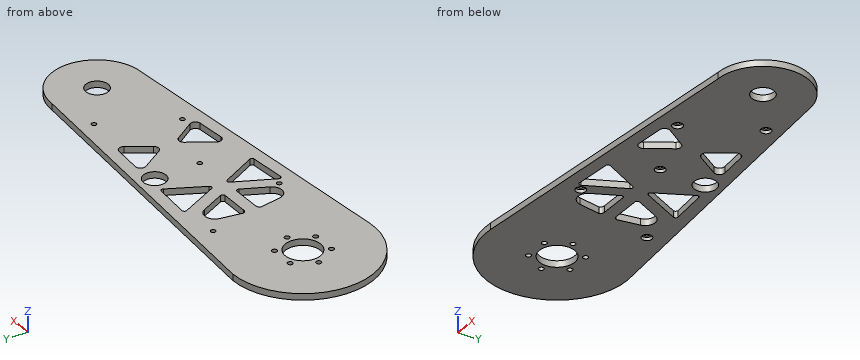
from build123d import *

# Parameters (mm, degrees)
SKETCH1_R              = 14.29385
SKETCH1_R_2            = 11.115
SKETCH1_R_3            = 11.1125
BOSS_EXTRUDE1_DEPTH    = 6.35
CROQUIS1_R             = 2.38125
CORTAR_EXTRUIR1_DEPTH  = 50
CROQUIS6_R             = 2.38125
CORTAR_EXTRUIR6_DEPTH  = 10
CROQUIS8_R             = 17.5
CORTAR_EXTRUIR8_DEPTH  = 10
CROQUIS9_R             = 2.5527
CORTAR_EXTRUIR9_DEPTH  = 10
CROQUIS5_R             = 2.38125
CORTAR_EXTRUIR5_DEPTH  = 10
CROQUIS10_R            = 5
CORTAR_EXTRUIR10_DEPTH = 3.18


with BuildPart() as part:
    # Sketch1 → Boss-Extrude1 (new body)
    with BuildSketch(Plane.XY):
        with BuildLine():
            Line((0, 70), (310, 45))
            ThreePointArc((310, 45), (355, 0), (310, -45))
            Line((310, -45), (5.171398252, -69.808714643))
            ThreePointArc((5.171398252, -69.808714643), (-69.952162315, -2.587467389), (0, 70))
        make_face()
        Circle(SKETCH1_R, mode=Mode.SUBTRACT)
        with Locations((310, 0)):
            Circle(SKETCH1_R_2, mode=Mode.SUBTRACT)
        with Locations((162.878542763, 40)):
            Circle(SKETCH1_R_3, mode=Mode.SUBTRACT)
        with BuildLine():
            Line((107.898974887, 49.259511156), (143.314248041, 46.40344074))
            ThreePointArc((143.314248041, 46.40344074), (145.093535791, 45.259647961), (145.131116366, 43.144768645))
            Line((145.131116366, 43.144768645), (127.657910713, 9.007596386))
            ThreePointArc((127.657910713, 9.007596386), (125.636568061, 7.786360797), (123.64194899, 9.050772613))
            Line((123.64194899, 9.050772613), (105.699881489, 46.044015288))
            ThreePointArc((105.699881489, 46.044015288), (105.866657482, 48.289689684), (107.898974887, 49.259511156))
        make_face(mode=Mode.SUBTRACT)
        with BuildLine():
            Line((80.397390769, 6), (108.202865744, 6))
            ThreePointArc((108.202865744, 6), (110.104277592, 7.052601687), (110.221605239, 9.222756416))
            Line((110.221605239, 9.222756416), (98.78989754, 32.792834786))
            ThreePointArc((98.78989754, 32.792834786), (88.404337676, 38.332134222), (79.941746192, 30.151166228))
            Line((79.941746192, 30.151166228), (76.136119631, 8.384360826))
            ThreePointArc((76.136119631, 8.384360826), (77.955894903, 6.636618521), (80.397390769, 6))
        make_face(mode=Mode.SUBTRACT)
        with BuildLine():
            Line((219.623774494, 32.810522613), (206.130928429, 12.417497436))
            ThreePointArc((206.130928429, 12.417497436), (201.919524559, 10.176643248), (197.745901529, 12.48710226))
            Line((197.745901529, 12.48710226), (183.296864227, 35.133505128))
            ThreePointArc((183.296864227, 35.133505128), (183.227765467, 40.400743015), (187.913912204, 42.80669363))
            Line((187.913912204, 42.80669363), (215.855795571, 40.553315939))
            ThreePointArc((215.855795571, 40.553315939), (219.949772588, 37.757395035), (219.623774494, 32.810522613))
        make_face(mode=Mode.SUBTRACT)
        with BuildLine():
            Line((98.78989754, -32.792834786), (110.221605239, -9.222756416))
            ThreePointArc((110.221605239, -9.222756416), (110.104277592, -7.052601687), (108.202865744, -6))
            Line((108.202865744, -6), (80.397390769, -6))
            ThreePointArc((80.397390769, -6), (77.955894903, -6.636618521), (76.136119631, -8.384360826))
            Line((76.136119631, -8.384360826), (79.941746192, -30.151166228))
            ThreePointArc((79.941746192, -30.151166228), (88.404337676, -38.332134222), (98.78989754, -32.792834786))
        make_face(mode=Mode.SUBTRACT)
        with BuildLine():
            Line((187.913912204, -42.80669363), (215.855795571, -40.553315939))
            ThreePointArc((215.855795571, -40.553315939), (219.949772588, -37.757395035), (219.623774494, -32.810522613))
            Line((219.623774494, -32.810522613), (206.130928429, -12.417497436))
            ThreePointArc((206.130928429, -12.417497436), (201.919524559, -10.176643248), (197.745901529, -12.48710226))
            Line((197.745901529, -12.48710226), (183.296864227, -35.133505128))
            ThreePointArc((183.296864227, -35.133505128), (183.227765467, -40.400743015), (187.913912204, -42.80669363))
        make_face(mode=Mode.SUBTRACT)
        with BuildLine():
            Line((123.64194899, -9.050772613), (105.699881489, -46.044015288))
            ThreePointArc((105.699881489, -46.044015288), (105.866657482, -48.289689684), (107.898974887, -49.259511156))
            Line((107.898974887, -49.259511156), (143.314248041, -46.40344074))
            ThreePointArc((143.314248041, -46.40344074), (145.093535791, -45.259647961), (145.131116366, -43.144768645))
            Line((145.131116366, -43.144768645), (127.657910713, -9.007596386))
            ThreePointArc((127.657910713, -9.007596386), (125.636568061, -7.786360797), (123.64194899, -9.050772613))
        make_face(mode=Mode.SUBTRACT)
    extrude(amount=BOSS_EXTRUDE1_DEPTH)

    # Croquis1 → Cortar-Extruir1 (cut)
    with BuildSketch(Plane.XY.offset(6.35)):
        with Locations((99.417366651, -42.272966779)):
            Circle(CROQUIS1_R)
        with Locations((229.299162877, -31.702435007)):
            Circle(CROQUIS1_R)
    extrude(amount=-CORTAR_EXTRUIR1_DEPTH, mode=Mode.SUBTRACT)

    # Croquis6 → Cortar-Extruir6 (cut)
    with BuildSketch(Plane.XY.offset(6.35)):
        with Locations((66.263169386, 45.68611009)):
            Circle(CROQUIS6_R)
        with Locations((263.293381054, 34.027262471)):
            Circle(CROQUIS6_R)
    extrude(amount=-CORTAR_EXTRUIR6_DEPTH, mode=Mode.SUBTRACT)

    # Croquis8 → Cortar-Extruir8 (cut)
    with BuildSketch(Plane.XY.offset(6.35)):
        Circle(CROQUIS8_R)
    extrude(amount=-CORTAR_EXTRUIR8_DEPTH, mode=Mode.SUBTRACT)

    # Croquis9 → Cortar-Extruir9 (cut)
    with BuildSketch(Plane(origin=(0, 0, 0), x_dir=(-1, 0, 0), z_dir=(0, 0, -1))):
        with Locations((23.8125, 0)):
            Circle(CROQUIS9_R)
        with Locations((11.90625, -20.622229928)):
            Circle(CROQUIS9_R)
        with Locations((-11.90625, -20.622229928)):
            Circle(CROQUIS9_R)
        with Locations((-23.8125, 0)):
            Circle(CROQUIS9_R)
        with Locations((-11.90625, 20.622229928)):
            Circle(CROQUIS9_R)
        with Locations((11.90625, 20.622229928)):
            Circle(CROQUIS9_R)
    extrude(amount=-CORTAR_EXTRUIR9_DEPTH, mode=Mode.SUBTRACT)

    # Croquis5 → Cortar-Extruir5 (cut)
    with BuildSketch(Plane.XY.offset(6.35)):
        with Locations((162.878542763, -5)):
            Circle(CROQUIS5_R)
    extrude(amount=-CORTAR_EXTRUIR5_DEPTH, mode=Mode.SUBTRACT)

    # Croquis10 → Cortar-Extruir10 (cut)
    with BuildSketch(Plane(origin=(0, 0, 0), x_dir=(-1, 0, 0), z_dir=(0, 0, -1))):
        with Locations((-263.293381054, 34.027262471)):
            Circle(CROQUIS10_R)
        with Locations((-66.263169386, 45.68611009)):
            Circle(CROQUIS10_R)
        with Locations((-229.299162877, -31.702435007)):
            Circle(CROQUIS10_R)
        with Locations((-99.417366651, -42.272966779)):
            Circle(CROQUIS10_R)
        with Locations((-162.878542763, -5)):
            Circle(CROQUIS10_R)
    extrude(amount=-CORTAR_EXTRUIR10_DEPTH, mode=Mode.SUBTRACT)


solid = part.part
Here's how the part is built. I have some questions about the finished solid (model axes, mm). Coordinates: 2 decimals unless noted, no trailing zeros. Order: outer loops, then holes, each group sorted by start corner. A loop starts at its lowest first (then second) coordinate and runs counter-clockwise, first axis right, second up. Notation, with made-up numbers: M 40,16.5 L 84,16.5 A17 cw 84,39.5 Z; hole C 79,14.25 d4. An arc over 180 degrees is marked long. Answer as CSV lines item,"result". Start each with the question number.
1. I need wall thicknesses on line 1 (Y direction, x = 167, z = 1.25); line 2 (X direction, y = -32.5, z = 4); line 3 (X direction, y = -31.5, z = 3). Which ranges of each line are inside material? Lowest first, please. Write a range as [from, to].
2. I want a section at A-A, the plane z = 1.75. Count the separate pieces of the cut face and the enclosed holes in it, and give its area (3 significant figures).
3. I want a section at B-B, the plane y = -60. Write out the boundary of the cut face in (x, z), and give its area (3 significant figures).
4. For pin 1 (1.5 mm diameter, centred on x = 300, z = 5, fed in from -Y); pin 2 (3 mm diameter, centred on y = -33, z = 4, fed in from +X); pin 3 (1.5 mm diameter, centred on x = 61.5, z = 4.5, fed in from +Y), each with a flat end and sliding along its axis, tell me the tip position at first contact or that it passes through.
Recorded:
1,line 1,"y = [-56.64, -7.83], [-2.17, 29.68], [50.32, 56.53]"
1,line 2,"x = [-62, 80.66], [98.93, 112.27], [139.68, 184.98], [219.42, 227.06], [231.54, 341.12]"
1,line 3,"x = [-62.51, 80.28], [99.42, 112.75], [139.17, 185.62], [218.76, 224.3], [234.3, 342.14]"
2,separate pieces,"1"
2,enclosed holes,"20"
2,area,"39,400 mm2"
3,outline,"M -36.06,0 L 125.69,0 L 125.69,6.35 L -36.06,6.35 Z"
3,area,"1,030 mm2"
4,pin 1,"stops at y = -45.87"
4,pin 2,"stops at x = 342.14"
4,pin 3,"stops at y = 65.1"
